Autodesk Inventor part; units mm, degrees
ref_plane "YZ Plane" through (0, 0, 0) normal (1, 0, 0) x (0, 1, 0)
ref_plane "XZ Plane" through (0, 0, 0) normal (0, 1, 0) x (-1, 0, 0)
ref_plane "XY Plane" through (0, 0, 0) normal (0, 0, 1) x (1, 0, 0)
sketch "Sketch1" plane through (0, 0, 0) normal (0, 0, 1) x (1, 0, 0)
  line L0 (0, 0) -> (220, 0) construction
  line L1 (220, 0) -> (220, 9) construction
  line L2 (220, 9) -> (0, 9) construction
  line L3 (0, 9) -> (0, 0) construction
  line L4 (0, 9) -> (90.94, 295.0593) construction
  line L5 (129.06, 295.0593) -> (220, 9) construction
  circle A0 centre (110, 289) radius 11 construction
  line L6 (96.1101, 281.616) -> (103.5522, 305.0259) construction
  arc A1 (129.06, 295.0593) -> (90.94, 295.0593) centre (110, 289) ccw construction
  line L7 (99, 275.5567) -> (99, 269.1274) construction
  line L8 (110, 289) -> (110, 143) construction
  line L9 (130, 289) -> (130, 143)
  line L10 (90, 143) -> (90, 289)
  arc A2 (130, 289) -> (90, 289) centre (110, 289) ccw
  arc A3 (90, 143) -> (130, 143) centre (110, 143) ccw
  line L11 (292.2692, 143) -> (292.2692, 247) construction
  line L12 (312.2692, 143) -> (312.2692, 247) construction
  line L13 (272.2692, 247) -> (272.2692, 143) construction
  arc A4 (272.2692, 143) -> (312.2692, 143) centre (292.2692, 143) ccw construction
  arc A5 (312.2692, 247) -> (272.2692, 247) centre (292.2692, 247) ccw construction
  arc A6 (90, 289) -> (130, 289) centre (110, 289) ccw construction
  line L14 (101.1908, 269) -> (118.8092, 269) construction
  line L15 (211.2941, 267) -> (373.2442, 267) construction
  line L16 (211.2941, 143) -> (373.2442, 143) construction
  line L17 (292.2692, 143) -> (292.2692, 39) construction
  line L18 (312.2692, 143) -> (312.2692, 39) construction
  line L19 (272.2692, 39) -> (272.2692, 143) construction
  arc A7 (312.2692, 143) -> (272.2692, 143) centre (292.2692, 143) ccw construction
  arc A8 (272.2692, 39) -> (312.2692, 39) centre (292.2692, 39) ccw construction
  line L20 (211.2941, 19) -> (373.2442, 19) construction
  circle A9 centre (110, 289) radius 11
  circle A10 centre (110, 143) radius 11
  point P0 (110, 0)
  point P1 (110, 216)
  point P2 (110, 309)
  point P3 (292.2692, 195)
  point P4 (110, 269)
  point P5 (110, 269)
  point P6 (292.2692, 267)
  dimension "d0" = 9
  dimension "d1" = 220
  dimension "d2" = 22
  dimension "d3" = 280
  dimension "d4" = 9
  dimension "d7" = 40
  dimension "d8" = 40
  dimension "pendgap" = 2
  dimension "abovethefloor" = 10
  dimension "d11" = 104
  dimension "d12" = 146
  dimension "d14" = 22
extrude "Extrusion2" add sketch "Sketch1" along normal blind 8
properties part number "FirstPendulum"
Work out the finished part from the listing and answer in its coordinate system (mm). Give positions to 0.01 mm unless a question says otherwise; leave off trailing zeros. Loops run counter-clockwise (first coordinate to the right, second up) from the corner with the lowest first, then second, coordinate; pieces in that order, holes last. Notation, with made-up numbers: (-26, 46.5) - (-1, 46.5) arc R17 ccw to (-1, 52.5) - close; hole circle Ø11 at (57.25, 7.25). An arc over 180 degrees is marked (long way). Answer in a Markdown table with one row per item. Add a question column.
Q1. The part is cut by section A-A (x = 110). Determine the outline of the cut face in (y, z), and give its area (3 significant figures).
Q2. Each of these flat-tipped pins is pushed along its axis until it touches: P1, Ø3, axis at x = 106, z = 4, coming from the +Y side; P2, Ø2, axis at x = 105, z = 5.5, coming from the -Y side. Where does it stop, or does it pass through?
Q3. The part is cut by section D-D (x = 119). Determine the outline of the cut face in (y, z), and give its area (3 significant figures).
Q4. Determine the mould class of faces 1 (the flat face through (90, 215, 4)), 2 (the cylindrical face through (101.89, 281.57, 3.94)), 3 (the cylindrical face through (110, 309, 4)) for opening direction Y: released by +Y, released by -Y, zero draft, split by the parting line, or undercut.
Q5. The part is cut by section B-B (y = 135). Determine the outline of the cut face in (x, z).
Q6. The part is cut by section C-C (z = 2.5). Determine the outline of the cut face in (x, y).
Q7. Consider line 1 along Y through (x, z) = (110, 3.25); line 2 along Y through (x, z) = (119, 5.5); line 3 along Y through (x, z) = (123.5, 1.75). Determine where each line is inside the solid, lowest interval first.
Solution:
| question | item | result |
|---|---|---|
| 1 | outline | (123, 0) - (132, 0) - (132, 8) - (123, 8) - close; (154, 0) - (278, 0) - (278, 8) - (154, 8) - close; (300, 0) - (309, 0) - (309, 8) - (300, 8) - close |
| 1 | area | 1,140 mm² |
| 2 | P1 | stops at y = 308.84 |
| 2 | P2 | stops at y = 123.4 |
| 3 | outline | (125.14, 0) - (136.68, 0) - (136.68, 8) - (125.14, 8) - close; (149.32, 0) - (282.68, 0) - (282.68, 8) - (149.32, 8) - close; (295.32, 0) - (306.86, 0) - (306.86, 8) - (295.32, 8) - close |
| 3 | area | 1,250 mm² |
| 4 | face 1 | zero draft |
| 4 | face 2 | undercut |
| 4 | face 3 | released by +Y |
| 5 | outline | (91.67, 0) - (102.45, 0) - (102.45, 8) - (91.67, 8) - close; (117.55, 0) - (128.33, 0) - (128.33, 8) - (117.55, 8) - close |
| 6 | outline | (90, 143) arc R20 ccw to (130, 143) - (130, 289) arc R20 ccw to (90, 289) - close; hole circle Ø22 at (110, 143); hole circle Ø22 at (110, 289) |
| 7 | line 1 | y = 123 to 132, 154 to 278, 300 to 309 |
| 7 | line 2 | y = 125.14 to 136.68, 149.32 to 282.68, 295.32 to 306.86 |
| 7 | line 3 | y = 128.24 to 303.76 |
